Design review of the part built by this model. Coordinates are the model's own, in mm. Face numbers are marked on the shaded views. A direction names the side the tool comes from. Round coordinates to 2 decimals unless told otherwise and drop trailing zeros. Order: outer loops, then holes, each group sorted by start corner. A loop starts at its lowest first (then second) coordinate and runs counter-clockwise, first axis right, second up. Notation, with made-up numbers: (10.25, 1.25) - (24.25, 1.25) arc R17 cw to (24.25, 15.25) - close; hole circle Ø5 at (80.25, 61.25). An arc over 180 degrees is marked (long way). Write item = value, one per line.
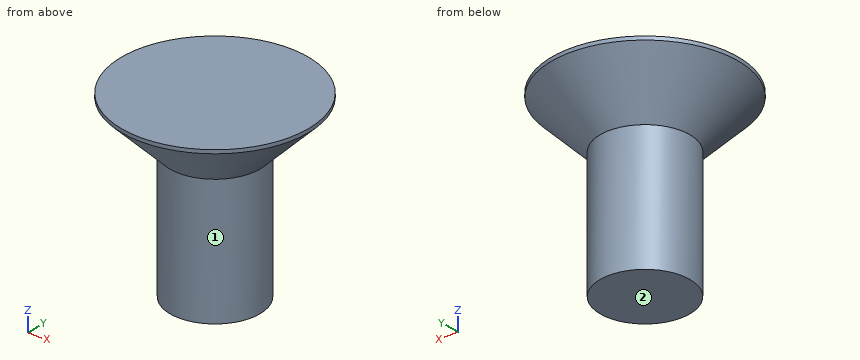
Autodesk Inventor part; units mm, degrees
ref_plane "YZ Plane" through (0, 0, 0) normal (1, 0, 0) x (0, 1, 0)
ref_plane "XZ Plane" through (0, 0, 0) normal (0, 1, 0) x (-1, 0, 0)
ref_plane "XY Plane" through (0, 0, 0) normal (0, 0, 1) x (1, 0, 0)
sketch "スケッチ1" plane through (0, 0, 0) normal (0, 0, 1) x (1, 0, 0)
  circle A0 centre (0, 0) radius 1.25
  dimension "d0" = 2.5
extrude "押し出し1" add sketch "スケッチ1" along normal blind 5
sketch "スケッチ2" plane through (0, 0, 5) normal (0, 0, 1) x (1, 0, 0)
  circle A0 centre (0, 0) radius 2.6
  dimension "d3" = 5.2
extrude "押し出し2" add sketch "スケッチ2" against normal blind 1.45
thread "ねじ1"
chamfer "面取り1" distance 1.35 angle 45 1 edges at (-2.6, 0, 3.55)
properties part number "ネジ皿m2.6,5" material "鋼、高強度、低合金"
1) We need section D-D on z = 4.45. Write out the cut boundary in (x, y).
Findings:
outline = circle Ø4.3 at (0, 0)
2) To check wall thickness, follow L1, parallel to Z at x = -1.2, y = 0.6; L2, parallel to Z at x = 0.6, y = -1.8; L3, parallel to X at y = -0.3, z = 2.15. State the ranges of each line that lie inside material, in increasing order. Write a range as from..to.
Findings:
L1 = 3.64..5
L2 = 4.2..5
L3 = -1.21..1.21
3) We need section C-C on z = 2. Write out the cut boundary in (x, y).
Findings:
outline = circle Ø2.5 at (0, 0)
4) Clearance check with a flat-ended pin moving along its axis: pin 1 Ø1.5 at (y, z) = (-2, 4.5) entering from -X. State where the tip first meets the part, or that it passes through.
Findings:
pin_1 = -2.21
5) For the marked faces 1 and 2, list the 3-axis set-ups (+Z, -Z, +X, -X, +Y, -Y) from which the entire face can be reached by the end or side of a thin tool; tool diameter is ignored.
Findings:
face_1 = -Z
face_2 = -Z, +X, -X, +Y, -Y
